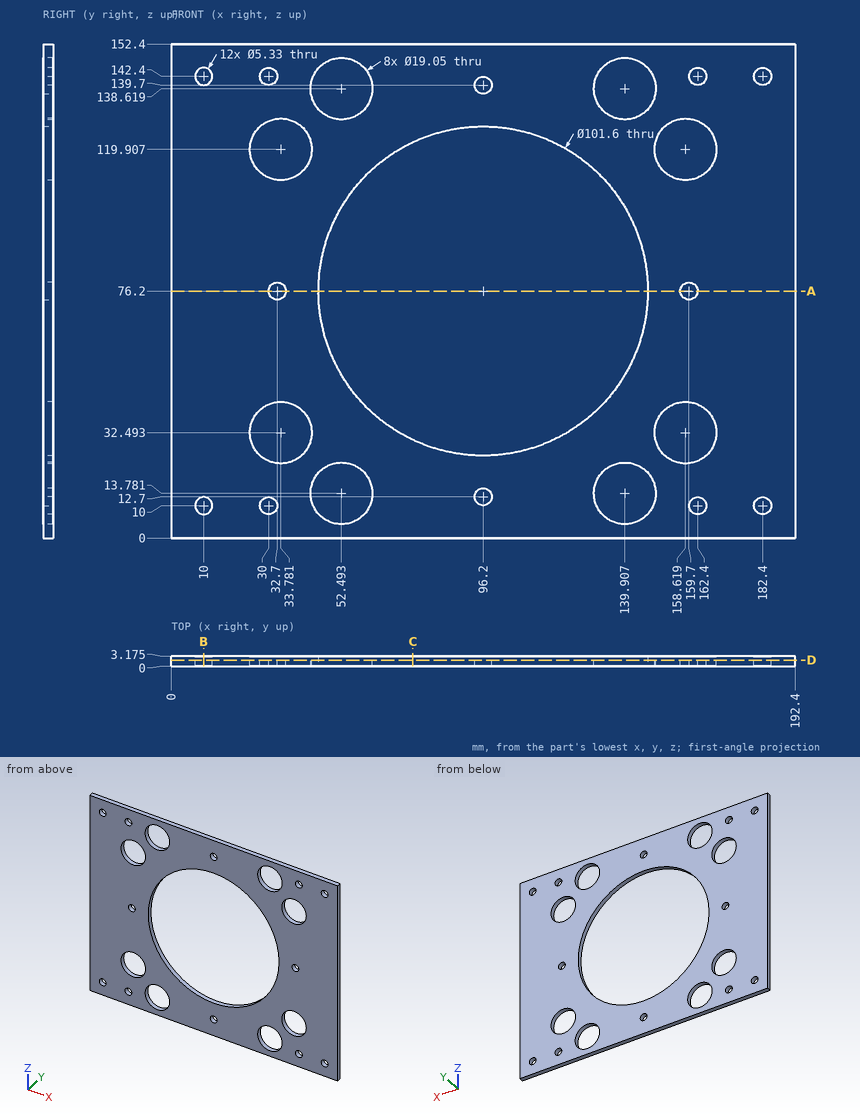
Can you work these out from the drawing? Everything is in mm from the part's minimum corner. Give positions to 0.01 mm unless a question says otherwise; leave off trailing zeros. Loops run counter-clockwise (first coordinate to the right, second up) from the corner with the lowest first, then second, coordinate; pieces in that order, holes last. Notation, with made-up numbers: (33.25, 62) -> (47.25, 62) arc R11 cw to (47.25, 83) -> close; hole circle Ø1 at (83.5, 67.25). An arc over 180 degrees is marked (long way). Put each result on its own line as item: value.
(1) I'm going to push a flat-ended pin straight in: pin 1 Ø6 at (x, z) = (96.2, 12.7) entering from -Y. Where does the tip first touch, or does it pass through?
Computed:
pin 1: y = 0
(2) Imagine slicing it at C-C on x = 74.5. Write out the boundary of the cut face in (y, z) (1 decimal).
Computed:
outline: (0, 0) -> (3.2, 0) -> (3.2, 30.3) -> (0, 30.3) -> close; (0, 122.1) -> (3.2, 122.1) -> (3.2, 152.4) -> (0, 152.4) -> close
(3) Please list where these lines run through material, in increasing order: probe 1 along X at (y, z) = (1.55, 76.2) (1 decimal); probe 2 along Z at (x, y) = (10, 1.7) (1 decimal); probe 3 along X at (y, z) = (1.8, 120.5) (1 decimal). Write a range as [from, to].
Computed:
probe 1: [0, 30], [35.4, 45.4], [147, 157], [162.4, 192.4]
probe 2: [0, 7.3], [12.7, 139.7], [145.1, 152.4]
probe 3: [0, 24.3], [43.3, 71.3], [121.1, 149.1], [168.1, 192.4]
(4) Imagine slicing it at A-A on z = 76.2. Write out the boundary of the cut face in (x, y) (1 decimal).
Computed:
outline: (0, 0) -> (30, 0) -> (30, 3.2) -> (0, 3.2) -> close; (35.4, 0) -> (45.4, 0) -> (45.4, 3.2) -> (35.4, 3.2) -> close; (147, 0) -> (157, 0) -> (157, 3.2) -> (147, 3.2) -> close; (162.4, 0) -> (192.4, 0) -> (192.4, 3.2) -> (162.4, 3.2) -> close
(5) Imagine slicing it at D-D on y = 1.9. State how many separate pieces and enclosed holes the cut face has, plus the area to 3 significant figures.
Computed:
separate pieces: 1
enclosed holes: 21
area: 18,700 mm^2
(6) Imagine slicing it at B-B on x = 10. Write out the boundary of the cut face in (y, z) (1 decimal), plus the area to 3 significant figures.
Computed:
outline: (0, 0) -> (3.2, 0) -> (3.2, 7.3) -> (0, 7.3) -> close; (0, 12.7) -> (3.2, 12.7) -> (3.2, 139.7) -> (0, 139.7) -> close; (0, 145.1) -> (3.2, 145.1) -> (3.2, 152.4) -> (0, 152.4) -> close
area: 450 mm^2
